Input: part model. Units: mm. Frame: model coordinates. A direction names the side the tool comes from. Coordinates: 2 decimals unless noted, no trailing zeros. Order: outer loops, then holes, each group sorted by start corner. A loop starts at its lowest first (then second) coordinate and runs counter-clockwise, first axis right, second up.
from build123d import *

# Parameters (mm, degrees)
EXTRUDE_THIN1_DEPTH = 285.75
FILLET1_R           = 1.016


with BuildPart() as part:
    # Sketch1 → Extrude-Thin1 (new body)
    with BuildSketch(Plane.XY):
        with BuildLine():
            Line((-0.396875, -9.555854473), (0, -14.318354473))
            Line((0, -14.318354473), (-7.9375, -14.318354473))
            Line((-7.9375, -14.318354473), (-7.9375, -12.730854473))
            ThreePointArc((-7.9375, -12.730854473), (-12.904112533, -12.290327979), (-17.543767938, -10.46415675))
            ThreePointArc((-17.543767938, -10.46415675), (-22.883426301, -8.487890863), (-28.575, -8.334375))
            Line((-28.575, -8.334375), (-28.575, -5.159375))
            Line((-28.575, -5.159375), (-9.525, -5.159375))
            Line((-9.525, -5.159375), (-9.525, 5.159375))
            Line((-9.525, 5.159375), (-28.575, 5.159375))
            Line((-28.575, 5.159375), (-28.575, 8.334375))
            ThreePointArc((-28.575, 8.334375), (-22.883426301, 8.487890863), (-17.543767938, 10.46415675))
            ThreePointArc((-17.543767938, 10.46415675), (-12.515637367, 12.377330284), (-7.14375, 12.669145527))
            Line((-7.14375, 12.669145527), (-7.14375, 14.256645527))
            Line((-7.14375, 14.256645527), (0, 14.256645527))
            Line((0, 14.256645527), (-0.396875, 9.494145527))
            Line((-0.396875, 9.494145527), (-1.40936549, 9.578519735))
            Line((-1.40936549, 9.578519735), (-1.104188341, 13.240645527))
            Line((-1.104188341, 13.240645527), (-6.12775, 13.240645527))
            Line((-6.12775, 13.240645527), (-6.12775, 11.50678851))
            ThreePointArc((-6.12775, 11.50678851), (-11.751151598, 11.490941353), (-17.040496255, 9.581561932))
            ThreePointArc((-17.040496255, 9.581561932), (-22.1225879, 7.60931063), (-27.559, 7.205758691))
            Line((-27.559, 7.205758691), (-27.559, 6.175375))
            Line((-27.559, 6.175375), (-8.509, 6.175375))
            Line((-8.509, 6.175375), (-8.509, -6.175375))
            Line((-8.509, -6.175375), (-27.559, -6.175375))
            Line((-27.559, -6.175375), (-27.559, -7.205758691))
            ThreePointArc((-27.559, -7.205758691), (-22.1225879, -7.60931063), (-17.040496255, -9.581561932))
            ThreePointArc((-17.040496255, -9.581561932), (-12.145263139, -11.416445859), (-6.9215, -11.622370501))
            Line((-6.9215, -11.622370501), (-6.9215, -13.302354473))
            Line((-6.9215, -13.302354473), (-1.104188341, -13.302354473))
            Line((-1.104188341, -13.302354473), (-1.40936549, -9.64022868))
            Line((-1.40936549, -9.64022868), (-0.396875, -9.555854473))
        make_face()
    extrude(amount=-EXTRUDE_THIN1_DEPTH)

    # Fillet1
    fillet1_edges = [part.edges().sort_by_distance(p)[0] for p in [
        (-7.9375, -14.318354473, -142.875),
        (-28.575, -8.334375, -142.875),
        (-28.575, -5.159375, -142.875),
        (-28.575, 5.159375, -142.875),
        (-28.575, 8.334375, -142.875),
        (-7.14375, 14.256645527, -142.875),
        (-6.12775, 11.50678851, -142.875),
        (-8.509, 6.175375, -142.875),
        (-8.509, -6.175375, -142.875),
        (-6.9215, -11.622370501, -142.875),
    ]]
    fillet(fillet1_edges, radius=FILLET1_R)


solid = part.part
Item 1: Cut plane B-B on y = -0.25. Return loops of the section in (x, z) (3 decimals), then the cut area to 3 significant figures.
Response values:
outline: (-9.525, -285.75) - (-8.509, -285.75) - (-8.509, 0) - (-9.525, 0) - close
area: 290 mm2
Item 2: Pin query (flat end, axial travel): pin 1 Ø5.5 at (x, z) = (-19, -158) entering from +Y; pin 2 Ø11.5 at (y, z) = (-0.5, -90.5) entering from -X (3 decimals); pin 3 Ø4 at (y, z) = (-10, -200.5) entering from +X; pin 4 Ø5 at (y, z) = (-2.5, -118) entering from +X. Return the tip coordinate at first contact, or that it passes through.
Response values:
pin 1: stops at y = 11.13
pin 2: stops at x = -28.575
pin 3: stops at x = -0.19
pin 4: stops at x = -8.51
Item 3: Draft query along X for faces 5 (the face through (-4, 13.241, -141)), 6 (the face through (-0.196, 11.909, -140.875)), 7 (the face through (-14.22, 5.33, 0)), 8 (the face through (-9.525, 0, -141)). Return one class per face: pulls with the +X half, pulls with the -X half, needs draft (parallel to the pull), parting line crosses it, or undercut.
Response values:
face 5: undercut
face 6: pulls with the +X half
face 7: needs draft
face 8: pulls with the -X half
Item 4: Ray query, probe 1 along Y at (x, z) = (-10, -170.5); probe 2 along Y at (x, z) = (-25.5, -167); probe 3 along Y at (x, z) = (-4, -92). Return the intervals inside material, ascending.
Response values:
probe 1: y = -12.72 to -11.7, -6.18 to -5.16, 5.16 to 6.18, 11.7 to 12.72
probe 2: y = -8.19 to -7.17, -6.18 to -5.16, 5.16 to 6.18, 7.17 to 8.19
probe 3: y = -14.32 to -13.3, 13.24 to 14.26
Item 5: Cut plane A-A on x = -22. Return loops of the section in (y, z).
Response values:
outline: (-8.68, -285.75) - (-7.64, -285.75) - (-7.64, 0) - (-8.68, 0) - close; (-6.18, -285.75) - (-5.16, -285.75) - (-5.16, 0) - (-6.18, 0) - close; (5.16, -285.75) - (6.18, -285.75) - (6.18, 0) - (5.16, 0) - close; (7.64, -285.75) - (8.68, -285.75) - (8.68, 0) - (7.64, 0) - close
Item 6: Access query for faces 1 (the face through (-18, -6.175, -141)), 2 (the face through (-19, -5.159, -141)), 3 (the face through (-4, -13.302, -141)), 4 (the face through (-14.22, 5.33, -285.75)). Directions: +Z, -Z, +X, -X, +Y, -Y. A direction counts if a zero-diameter tool reaches every point of the face in a straight line with its end or side. Return the directions, or none.
Response values:
face 1: +Z, -Z, +X
face 2: +Z, -Z, -X
face 3: +Z, -Z
face 4: -Z, +X, -X, +Y, -Y
